```python
from build123d import *

# Parameters (mm, degrees)
F0_W     = 110
F0_H     = 20
F1_DEPTH = 3
F2_R     = 9
F3_W     = 3
F3_H     = 10
F4_DEPTH = 3


with BuildPart() as f1:
    # F0 (on Front) → F1 (new body)
    with BuildSketch(Plane.XZ):
        with Locations((59.607332, 10)):
            Rectangle(F0_W, F0_H)
    extrude(amount=F1_DEPTH)

    # F2
    f2_edges = [f1.edges().sort_by_distance(p)[0] for p in [
        (4.607332, -1.5, 20),
        (4.607332, -1.5, 0),
        (114.607332, -1.5, 20),
        (114.607332, -1.5, 0),
    ]]
    fillet(f2_edges, radius=F2_R)

    # F3 (on face) → F4 (cut)
    with BuildSketch(Plane.XZ.offset(3)):
        with Locations((99.883784, 15)):
            Rectangle(F3_W, F3_H)
    extrude(amount=-F4_DEPTH, mode=Mode.SUBTRACT)


solid = f1.part
```
Verification items for the finished model (mm, model axes). A direction names the side the tool comes from. Round coordinates to 2 decimals unless told otherwise and drop trailing zeros. Write each loop counter-clockwise with the first axis right and the second up, starting at its lowest first coordinate (ties: lowest second). Pieces come first, ordered by that corner, then holes.
1. Draft check along X on faces 1 (the flat face through (101.384, -2, 15)), 2 (the flat face through (4.607, -1, 10)), 3 (the flat face through (98.384, -2, 15)), 4 (the flat face through (55, -1, 20)). Enter one of: +X half, -X half, draft (parallel to the pull), parting line (faces both ways), or undercut.
2. Gauge pin test, flat ends, axial feed: P1, Ø1.5, axis at y = -1, z = 13, coming from the +X side; P2, Ø1.5, axis at x = 100.5, y = -1.5, coming from the +Z side; P3, Ø1.5, axis at y = -2, z = 15, coming from the -X side. Record the tip position at first contact, or that the pin passes through.
3. Section check B-B on z = 15. Enter the section's corners in (x, y).
4. Section check C-C on z = 2.5. Enter the section's corners in (x, y).
5. Section check A-A on y = -0.5. Enter the section's corners in (x, z), plus the area to 3 significant figures.
6. Scan lines: L1, parallel to X at y = -0.7, z = 19; L2, parallel to X at y = -1.8, z = 10.75; L3, parallel to Z at x = 99, y = -1.9. Record each from-to range of solid material in increasing order.
7. Access from +Z, -Z, +X, -X, +Y, -Y to the whole of each face (thin tool, end or side, straight path). Record for faces 5 (the flat face through (59, -3, 10)), 6 (the flat face through (100, -2, 10)).
Answer:
1. face 1: undercut
1. face 2: -X half
1. face 3: undercut
1. face 4: draft
2. P1: stops at x = 114.52
2. P2: stops at z = 10
2. P3: stops at x = 5.21
3. outline: (5.55, -3) - (98.38, -3) - (98.38, 0) - (5.55, 0) - close; (101.38, -3) - (113.67, -3) - (113.67, 0) - (101.38, 0) - close
4. outline: (7.38, -3) - (111.83, -3) - (111.83, 0) - (7.38, 0) - close
5. outline: (4.61, 9) arc R9 ccw to (13.61, 0) - (105.61, 0) arc R9 ccw to (114.61, 9) - (114.61, 11) arc R9 ccw to (105.61, 20) - (101.38, 20) - (101.38, 10) - (98.38, 10) - (98.38, 20) - (13.61, 20) arc R9 ccw to (4.61, 11) - close
5. area: 2,100 mm2
6. L1: x = 9.48 to 98.38, 101.38 to 109.73
6. L2: x = 4.61 to 98.38, 101.38 to 114.61
6. L3: z = 0 to 10
7. face 5: +Z, -Z, +X, -X, -Y
7. face 6: +Z, +Y, -Y
